Here's how the part is built. I have some questions about the finished solid (model axes, mm). A direction names the side the tool comes from. Round coordinates to 2 decimals unless told otherwise and drop trailing zeros. Order: outer loops, then holes, each group sorted by start corner. A loop starts at its lowest first (then second) coordinate and runs counter-clockwise, first axis right, second up. Notation, with made-up numbers: (24, 32) - (53, 32) arc R15 ccw to (53, 54) - close; hole circle Ø11 at (-36.5, 25). An arc over 180 degrees is marked (long way). One line per item, written item: value.
from build123d import *

# Parameters (mm, degrees)
SKETCH2_W          = 11.3
SKETCH2_H          = 1.6
CUT_EXTRUDE1_DEPTH = 2.8
CHAMFER1_SIZE      = 0.5


with BuildPart() as part:
    # Sketch1 → Revolve1 (revolve)
    with BuildSketch(Plane.XY):
        with BuildLine():
            Line((-1.4, 5.65), (-2.05, 5.65))
            Line((-2.05, 5.65), (-4.7, 3))
            Line((-4.7, 3), (-21.4, 3))
            Line((-21.4, 3), (-21.4, 0))
            Line((-21.4, 0), (0, 0))
            ThreePointArc((0, 0), (-0.355213526, 2.910433816), (-1.4, 5.65))
        make_face()
    revolve(axis=Axis((0, 0, 0), (-1, 0, 0)))

    # Sketch2 → Cut-Extrude1 (cut)
    with BuildSketch(Plane(origin=(0, 0, 0), x_dir=(0, 0, -1), z_dir=(1, 0, 0))):
        Rectangle(SKETCH2_W, SKETCH2_H)
    extrude(amount=-CUT_EXTRUDE1_DEPTH, mode=Mode.SUBTRACT)

    # Chamfer1
    chamfer1_edges = [part.edges().sort_by_distance(p)[0] for p in [
        (-21.4, -3, 0),
    ]]
    chamfer(chamfer1_edges, length=CHAMFER1_SIZE)


solid = part.part
Q1. If we section it at A-A, the plane y = 0: Please give me the cut outline in (x, z), then the cut area to 3 significant figures.
Results list:
outline: (-21.4, -2.5) - (-20.9, -3) - (-4.7, -3) - (-2.8, -4.9) - (-2.8, 4.9) - (-4.7, 3) - (-20.9, 3) - (-21.4, 2.5) - close
area: 115 mm²
Q2. Will these pins go through, and if not, where does the flat tip stop? pin 1 (2 mm diameter, centred on x = -13.5, y = 2.5, fed in from -Z); pin 2 (0.8 mm diameter, centred on y = 0.5, z = -2, fed in from +X).
Results list:
pin 1: z = -2.6
pin 2: x = -0.15
Q3. If we section it at B-B, the plane z = 0: Please give me the cut outline in (x, y).
Results list:
outline: (-21.4, -2.5) - (-20.9, -3) - (-4.7, -3) - (-2.05, -5.65) - (-1.4, -5.65) arc R12.1 ccw to (-0.03, -0.8) - (-2.8, -0.8) - (-2.8, 0.8) - (-0.03, 0.8) arc R12.1 ccw to (-1.4, 5.65) - (-2.05, 5.65) - (-4.7, 3) - (-20.9, 3) - (-21.4, 2.5) - close
Q4. If I drill on line 1 along X through (y, z) = (3.75, 3.5); line 2 along X through (y, z) = (1.75, -2.5); line 3 along Z through (x, y) = (-4.25, -2.25), over which ranges is the centre line in solid material (lowest first)?
Results list:
line 1: -2.57 to -1.14
line 2: -4.65 to -0.39
line 3: -2.62 to 2.62
Q5. We'd pull the mould along Y, two halves only. Please class faces 4 (the cylindrical face through (-1.73, -5.65, -0.11)), 5 (the flat face through (-21.4, 0, 0)), 6 (the flat face through (-2.8, 0, 0)), 7 (the conical face through (-4.571, -0.678, 3.054)): released by +Y, released by -Y, zero draft, split by the parting line, or undercut.
Results list:
face 4: released by -Y
face 5: zero draft
face 6: undercut
face 7: split by the parting line
Q6. If we section it at C-C, the plane x = -13: Please give me the cut outline in (y, z), then the cut area to 3 significant figures.
Results list:
outline: circle Ø6 at (0, 0)
area: 28.3 mm²
Q7. Which directions (+Z, -Z, +X, -X, +Y, -Y) give clear straight access to the entire face, cutting with the end or side of a thin tool? Please do faces 1 (the cylindrical face through (-13, -3, 0)), 2 (the cylindrical face through (-1.73, 5.65, 0.11)), 3 (the flat face through (-2, -0.8, 0)).
Results list:
face 1: -X
face 2: +X, -X, +Y
face 3: +Z, -Z, +X
